```python
from build123d import *

# Parameters (mm, degrees)
SKETCH1_R           = 9
BOSS_EXTRUDE1_DEPTH = 20
BOSS_EXTRUDE2_DEPTH = 60
SKETCH7_R           = 12
CUT_EXTRUDE1_DEPTH  = 150.255653211
SKETCH8_W           = 103.314171972
SKETCH8_H           = 30
CUT_EXTRUDE2_DEPTH  = 149.637983151
SKETCH10_W          = 10
SKETCH10_H          = 60
BOSS_EXTRUDE3_DEPTH = 65
CUT_EXTRUDE3_DEPTH  = 136.470476619


with BuildPart() as part:
    # Sketch1 → Boss-Extrude1 (new body)
    with BuildSketch(Plane(origin=(0, 0, 0), x_dir=(1, 0, 0), z_dir=(0, 1, 0))):
        with BuildLine():
            Line((-52.5, 45), (52.5, 45))
            ThreePointArc((52.5, 45), (66.642135624, 39.142135624), (72.5, 25))
            Line((72.5, 25), (72.5, -25))
            ThreePointArc((72.5, -25), (66.642135624, -39.142135624), (52.5, -45))
            Line((52.5, -45), (-52.5, -45))
            ThreePointArc((-52.5, -45), (-66.642135624, -39.142135624), (-72.5, -25))
            Line((-72.5, -25), (-72.5, 25))
            ThreePointArc((-72.5, 25), (-66.642135624, 39.142135624), (-52.5, 45))
        make_face()
        with Locations(Location((-52.5, 25, 0), (0, 0, 270))):
            Circle(SKETCH1_R, mode=Mode.SUBTRACT)
        with Locations(Location((-52.5, -25, 0), (0, 0, 270))):
            Circle(SKETCH1_R, mode=Mode.SUBTRACT)
    extrude(amount=-BOSS_EXTRUDE1_DEPTH)

    # Sketch2 → Boss-Extrude2 (add)
    with BuildSketch(Plane(origin=(0, 0, 0), x_dir=(1, 0, 0), z_dir=(0, 1, 0))):
        with BuildLine():
            Line((-7.5, 34), (42.5, 34))
            ThreePointArc((42.5, 34), (76.5, 0), (42.5, -34))
            Line((42.5, -34), (-7.5, -34))
            Line((-7.5, -34), (-7.5, 34))
        make_face()
    extrude(amount=BOSS_EXTRUDE2_DEPTH)

    # Loft1: read off the stored shape, not the designer's step
    # Loft1: loft between two sections, ruled curve by curve
    loft1_from = [
        Edge.make_bspline([(22.989923238, 100, -4.399648251), (31.789219739, 100, -43.419801775), (70.809373263, 100, -34.620505274), (62.010076762, 100, 4.399648251), (53.210780261, 100, 43.419801775), (14.190626737, 100, 34.620505274), (22.989923238, 100, -4.399648251)], [0, 0, 0, 0, 0.5, 0.5, 0.5, 1, 1, 1, 1], 3, [1, 0.333333333, 0.333333333, 1, 0.333333333, 0.333333333, 1]),
    ]
    loft1_to = [
        Edge.make_bspline([(10.620019024, 60, 11.818071457), (-13.01612389, 60, -51.941890495), (50.743838062, 60, -75.578033409), (74.379980976, 60, -11.818071457), (98.01612389, 60, 51.941890495), (34.256161938, 60, 75.578033409), (10.620019024, 60, 11.818071457)], [0, 0, 0, 0, 0.5, 0.5, 0.5, 1, 1, 1, 1], 3, [1, 0.333333333, 0.333333333, 1, 0.333333333, 0.333333333, 1]),
    ]
    loft1 = Solid(Shell([*[Face.make_surface_from_curves(loft1_from[k], loft1_to[k]) for k in range(1)], Face(Wire(loft1_from)), Face(Wire(loft1_to))]))
    add(loft1)

    # Sketch7 → Cut-Extrude1 (cut, through all)
    with BuildSketch(Plane(origin=(0, 100, 0), x_dir=(1, 0, 0), z_dir=(0, 1, 0))):
        with Locations(Location((42.5, 0, 0), (0, 0, 270))):
            Circle(SKETCH7_R)
    extrude(amount=-CUT_EXTRUDE1_DEPTH, mode=Mode.SUBTRACT)

    # Sketch8 → Cut-Extrude2 (cut, through all)
    with BuildSketch(Plane.XY.offset(34)):
        with Locations((64.157085986, 30)):
            Rectangle(SKETCH8_W, SKETCH8_H)
    extrude(amount=-CUT_EXTRUDE2_DEPTH, mode=Mode.SUBTRACT)

    # Sketch10 → Boss-Extrude3 (add, through all)
    with BuildSketch(Plane.ZY.offset(7.5)):
        with Locations((0, 30)):
            Rectangle(SKETCH10_W, SKETCH10_H)
    extrude(amount=BOSS_EXTRUDE3_DEPTH)

    # Sketch11 → Cut-Extrude3 (cut, through all)
    with BuildSketch(Plane.XY.offset(5)):
        Polygon((-7.5, 60), (-72.5, 0), (-72.5, 60), align=None)
    extrude(amount=-CUT_EXTRUDE3_DEPTH, mode=Mode.SUBTRACT)


solid = part.part
```
Design review of the part built by this model. Coordinates are the model's own, in mm. A direction names the side the tool comes from. Give positions to 0.01 mm unless a question says otherwise; leave off trailing zeros. Order: outer loops, then holes, each group sorted by start corner. A loop starts at its lowest first (then second) coordinate and runs counter-clockwise, first axis right, second up. Notation, with made-up numbers: M 10.25,79.5 L 21.25,79.5 A11 ccw 21.25,83.5 Z; hole C -10,-28 d8. An arc over 180 degrees is marked long. One line per question, with ' | ' between items. Start each with the question number.
Q1. For L1, parallel to X at y = -8, z = -25; L2, parallel to Y at x = 52, z = 9.5; L3, parallel to Y at x = 48, z = 41.5, list the stretches that pass through material, from the lowest coordinate up. Write a range as [from, to].
Q2. We need section B-B (z = 0). State how many separate pieces and enclosed holes the cut face has, plus the area to 3 significant figures.
Q3. The part is to be moulded in two halves that separate along Z. For faces 4 (the face through (30, 15, 0)), 5 (the face through (-49.797, -9.86, -16.416)), 6 (the face through (12, 30, 34)), say which applies: +Z half, -Z half, draft (parallel to the pull), parting line (faces both ways), or undercut.
Q4. We need section C-C (x = -20). Write out the cut boundary in (y, z), plus the area to 3 significant figures.
Q5. We need section A-A (x = -58.5). Write out the cut boundary in (y, z), plus the area to 3 significant figures.
Q6. For pin 1 Ø2 at (x, z) = (-13, -33.5) entering from +Y; pin 2 Ø19 at (x, z) = (47, -11) entering from -Y; pin 3 Ø6 at (x, z) = (-50, 20) entering from -Y; pin 4 Ø23 at (y, z) = (44.5, 19.5) entering from -X, all flat-tipped, find the tip position at first contact; note any pin that passes through.
Q7. Machinability: for faces 1 (the face through (74, 0, 0)), 2 (the face through (-7.5, 30, 20)), 3 (the face through (-32, 23, -5)), which of the approach directions +Z, -Z, +X, -X, +Y, -Y give a long, thin tool a straight path to every point of the face, cutting with its end or side? Answer none if there is none.
Returned:
1) L1: [-72.5, -61.5], [-43.5, 72.5] | L2: [-20, 15], [45, 100] | L3: [-20, 0]
2) separate pieces: 3 | enclosed holes: 0 | area: 7,910 mm2
3) face 4: draft | face 5: undercut | face 6: +Z half
4) outline: M -20,-45 L 0,-45 L 0,-5 L 48.46,-5 L 48.46,5 L 0,5 L 0,45 L -20,45 Z | area: 2,280 mm2
5) outline: M -20,-44.08 L 0,-44.08 L 0,-31.71 L -20,-31.71 Z; M -20,-18.29 L 0,-18.29 L 0,-5 L 12.92,-5 L 12.92,5 L 0,5 L 0,18.29 L -20,18.29 Z; M -20,31.71 L 0,31.71 L 0,44.08 L -20,44.08 Z | area: 1,360 mm2
6) pin 1: y = 0 | pin 2: y = -20 | pin 3: through | pin 4: x = -7.5
7) face 1: +Z, -Z, +X, -Y | face 2: +Z, -X, +Y | face 3: -Z, -X, +Y
